Autodesk Inventor part; units mm, degrees
ref_plane "YZ Plane" through (0, 0, 0) normal (1, 0, 0) x (0, 1, 0)
ref_plane "XZ Plane" through (0, 0, 0) normal (0, 1, 0) x (-1, 0, 0)
ref_plane "XY Plane" through (0, 0, 0) normal (0, 0, 1) x (1, 0, 0)
sketch "Sketch1" plane through (0, 0, 0) normal (0, 1, 0) x (-1, 0, 0)
  line L0 (20, 14.965) -> (-20, 14.965)
  line L1 (-20, 14.965) -> (-20, -14.965)
  line L2 (-20, -14.965) -> (20, -14.965)
  line L3 (20, -14.965) -> (20, 14.965)
  point P0 (0, 0)
  dimension "d0" = 29.93
  dimension "d1" = 40
  dimension "d2" = 20
  dimension "d3" = 14.965
extrude "Plate1" add sketch "Sketch1" along normal blind 1.5
sketch "Sketch2" plane through (-20, 0, -13.465) normal (0, 0, -1) x (-1, 0, 0)
  line L0 (-40, 0) -> (0, 0)
  line L1 (0, 0) -> (0, 43.5)
  line L2 (0, 43.5) -> (-40, 43.5)
  line L3 (-40, 43.5) -> (-40, 0)
edge flange "Flange1" height 43.5 angle 90 thickness 1.5 bend radius 0.31 thickness toward (0, 0, -1) relief tear relief width 1.5 relief depth 0.75 corner gap 0.31 corner form 0 edges at (0, 1.5, -14.965) (0, 1.5, 14.965) wall of the first edge with corners at (20, 0, -13.465) (-20, 0, -13.465) (-20, 43.5, -13.465) (20, 43.5, -13.465)
bend "Bend1"
corner "Corner1"
sketch "Sketch3" plane through (-20, 43.5, 14.965) normal (0, 0, 1) x (1, 0, 0)
  line L0 (0, 0) -> (40, 0)
  line L1 (0, -41.69) -> (0, 0)
  circle A0 centre (20, -10) radius 10
  line L2 (0, -28.19) -> (40, -28.19)
  line L3 (40, -28.19) -> (40, -38.19)
  line L4 (40, -38.19) -> (0, -38.19)
  line L5 (0, -38.19) -> (0, -28.19)
  line L6 (40, -28.19) -> (28.9876, -5.6156)
  line L7 (0, -28.19) -> (11.0124, -5.6156)
  line L8 (0, 0) -> (40, 0)
  line L9 (40, 0) -> (40, -35)
  line L10 (40, -35) -> (0, -35)
  line L11 (0, -35) -> (0, 0)
  point P0 (20, -43.5)
  point P1 (20, 0)
  point P2 (0, -28.19)
  point P3 (0, -35)
  point P4 (30, -10)
  dimension "d15" = 10
  dimension "d16" = 0
  dimension "d17" = 20
  dimension "d18" = 18.19
  dimension "d19" = 0
  dimension "d20" = 40
  dimension "d21" = 10
  dimension "d22" = 35
extrude "Extrusion1" cut sketch "Sketch3" against normal blind 35 contours L0 A0 L7 L1 | L0 L9 L6 A0
sketch "Sketch4" plane through (20, 1.81, -14.965) normal (0, 0, -1) x (-1, 0, 0)
  arc A0 (28.9876, 36.0744) -> (11.0124, 36.0744) centre (20, 31.69) ccw
  circle A1 centre (20, 31.69) radius 2.6
  circle A2 centre (13, 31.69) radius 1.05
  circle A3 centre (27, 31.69) radius 1.05
  circle A4 centre (20, 38.69) radius 1.05
  circle A5 centre (20, 24.69) radius 1.05
  point P0 (20, -1.81)
  dimension "d25" = 5.2
  dimension "d26" = 0
  dimension "d27" = 7
  dimension "d28" = 2.1
  dimension "d29" = 7
  dimension "d30" = 0
  dimension "d31" = 2.1
  dimension "d32" = 0
  dimension "d33" = 7
  dimension "d34" = 2.1
  dimension "d35" = 7
  dimension "d36" = 0
  dimension "d37" = 2.1
extrude "Extrusion2" cut sketch "Sketch4" against normal blind 1.5
sketch "Sketch5" plane through (-20, 1.81, 14.965) normal (0, 0, 1) x (1, 0, 0)
  arc A0 (28.9876, 36.0744) -> (11.0124, 36.0744) centre (20, 31.69) ccw
  circle A1 centre (20, 31.69) radius 2.5
  point P0 (20, -1.81)
  dimension "d40" = 5
extrude "Extrusion3" cut sketch "Sketch5" against normal blind 1.5
sketch "Sketch6" plane through (0, 1.5, 0) normal (0, 1, 0) x (1, 0, 0)
  circle A0 centre (-14, -10.155) radius 1.05
  circle A1 centre (-14, -0.75) radius 1.05
  circle A2 centre (-14, 8.655) radius 1.05
  circle A3 centre (14, -10.155) radius 1.05
  circle A4 centre (14, -0.75) radius 1.05
  circle A5 centre (14, 8.655) radius 1.05
  point P0 (0, 0)
hole "Hole1" at (14, 1.5, -8.655) at (14, 1.5, 0.75) at (14, 1.5, 10.155) at (-14, 1.5, 10.155) at (-14, 1.5, 0.75) at (-14, 1.5, -8.655) direction (0, -1, 0) diameter 2.1 depth 1.5
equation "\"d48\" = Thickness"
equation "\"d4\" = Thickness"
equation "\"d5\" = BendReliefWidth"
equation "\"d6\" = BendReliefDepth"
equation "\"d7\" = MinimumRemnant"
equation "\"d8\" = TransitionRadius"
equation "\"d11\" = BendRadius"
equation "\"d12\" = CornerReliefSize"
equation "\"d13\" = GapSize"
equation "\"d14\" = JacobiRadiusSize"
equation "\"BendReliefWidth\" = Thickness"
equation "\"BendReliefDepth\" = 0.5 * Thickness"
equation "\"CornerReliefSize\" = 4 * Thickness"
equation "\"MinimumRemnant\" = 2 * Thickness"
equation "\"TransitionRadius\" = BendRadius"
equation "\"JacobiRadiusSize\" = BendRadius"
equation "\"GapSize\" = Thickness"
properties part number "partpart" material "Aluminum 6061-AHC"
Check sheet for the modelled part. Datum: model origin and axes. Units: mm. A direction names the side the tool comes from. Round coordinates to 2 decimals unless told otherwise and drop trailing zeros. Loops run counter-clockwise (first coordinate to the right, second up) from the corner with the lowest first, then second, coordinate; pieces in that order, holes last. Notation, with made-up numbers: (34, 10) - (82, 10) arc R17 cw to (82, 14) - close; hole circle Ø6 at (-13, -17). An arc over 180 degrees is marked (long way). Answer as a JSON object with one key per item and string values. Group by question number.
Q1. Sectioned sample at C-C, the plane x = -7. Enter the section's corners in (y, z) (3 decimals).
Q2. Sectioned sample at B-B, the plane y = 13. Enter the section's corners in (x, z) (3 decimals).
Q3. Sectioned sample at D-D, the plane y = 26.5. Enter the section's corners in (x, z) (3 decimals).
Q4. Scan lines: line 1 along Z through (x, y) = (-2.5, 14) (3 decimals); line 2 along Y through (x, z) = (1, -1.5). Record each from-to range of solid material in increasing order. Write a range as [from, to].
Q5. Set-up check for faces 5 (the face through (-14.885, 0.74, -8.091)), 6 (the face through (0, 18, -13.465)), 7 (the face through (-1.4, 35.69, -14.23)): record each of +Z, -Z, +X, -X, +Y, -Y from which the full face is reachable in a straight line by a thin tool's end or side.
Q6. Sectioned sample at A-A, the plane z = 0.75. Enter the section's corners in (x, y).
Q7. Mould release check, pull along Z, two halves, no side actions. Record for faces 1 (the face through (-0.28, 0.544, -14.449)), 2 (the face through (0.28, 0.544, 14.449)), 3 (the face through (13.11, 0.74, 1.31)), 4 (the face through (-6.772, 32.475, -14.226)): released by +Z, released by -Z, zero draft, split by the parting line, or undercut.
Q8. Gauge pin test, flat ends, axial feed: P1, Ø2.5, axis at x = -14, z = 10.155, coming from the +Y side; P2, Ø1.9, axis at x = 7, y = 33.5, coming from the -Z side (3 decimals). Record the tip position at first contact, or that the pin passes through.
Solution:
{
 "1": {"outline": "(0, -13.155) arc R1.81 ccw to (1.81, -14.965) - (32.45, -14.965) - (32.45, -13.465) - (1.81, -13.465) arc R0.31 cw to (1.5, -13.155) - (1.5, 13.155) arc R0.31 cw to (1.81, 13.465) - (40.641, 13.465) - (40.641, 14.965) - (1.81, 14.965) arc R1.81 ccw to (0, 13.155) - close; (34.55, -14.965) - (40.641, -14.965) - (40.641, -13.465) - (34.55, -13.465) - close"},
 "2": {"outline": "(-20, -14.965) - (20, -14.965) - (20, -13.465) - (-20, -13.465) - close; (-20, 13.465) - (20, 13.465) - (20, 14.965) - (-20, 14.965) - close"},
 "3": {"outline": "(-14.541, -14.965) - (-1.05, -14.965) - (-1.05, -13.465) - (-14.541, -13.465) - close; (-14.541, 13.465) - (14.541, 13.465) - (14.541, 14.965) - (-14.541, 14.965) - close; (1.05, -14.965) - (14.541, -14.965) - (14.541, -13.465) - (1.05, -13.465) - close"},
 "4": {"line 1": "z = [-14.965, -13.465], [13.465, 14.965]", "line 2": "y = [0, 1.5]"},
 "5": {"face 5": "+Y, -Y", "face 6": "+X, -X, +Y", "face 7": "-Z"},
 "6": {"outline": "(-20, 0) - (-15.05, 0) - (-15.05, 1.5) - (-20, 1.5) - close; (-12.95, 0) - (12.95, 0) - (12.95, 1.5) - (-12.95, 1.5) - close; (15.05, 0) - (20, 0) - (20, 1.5) - (15.05, 1.5) - close"},
 "7": {"face 1": "released by -Z", "face 2": "released by +Z", "face 3": "undercut", "face 4": "zero draft"},
 "8": {"P1": "stops at y = 1.5", "P2": "stops at z = 13.465"}
}
